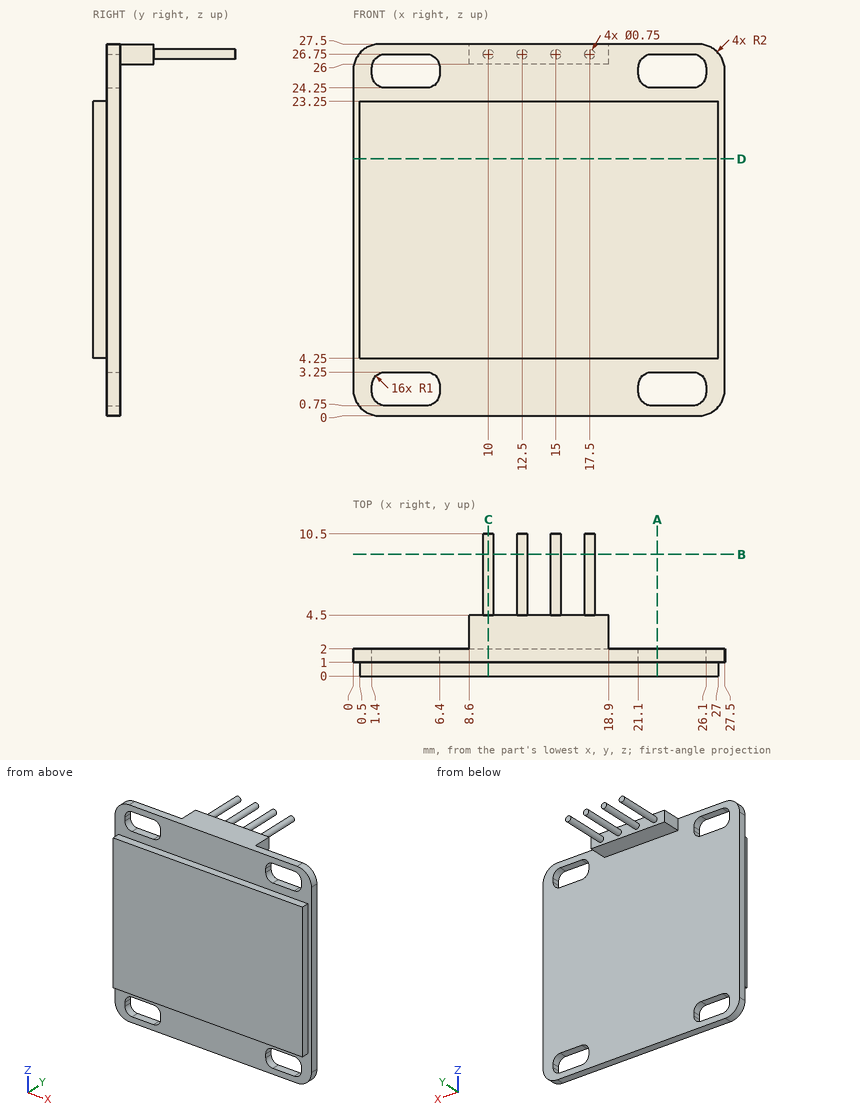
The drawing under review shows one solid part. Ordinate dimensions are in mm from its lowest x, y, z. Coordinates: 2 decimals unless noted, no trailing zeros. Write each loop counter-clockwise with the first axis right and the second up, starting at its lowest first coordinate (ties: lowest second). Pieces come first, ordered by that corner, then holes.
1) Insertion check: pin 1 (12 mm diameter, centred on x = 6.5, z = 3, fed in from +Y); pin 2 (0.5 mm diameter, centred on y = 0.5, z = 14, fed in from -X); pin 3 (0.5 mm diameter, centred on x = 11.5, y = 0.5, fed in from -Z). Each pin has a flat end and moves straight along its axis. Give the tip position at first contact, or say it passes through.
2) Add section A-A (x = 22.5). Write out the cut boundary in (y, z).
3) To check wall thickness, follow L1, parallel to Y at x = 19.75, z = 7; L2, parallel to Y at x = 20.5, z = 23.75; L3, parallel to Z at x = 8.75, y = 4.25. State the ranges of each line that lie inside material, in increasing order.
4) Add section D-D (z = 19). Write out the cut boundary in (x, y), plus the area to 3 significant figures.
5) Add section C-C (x = 10). Write out the cut boundary in (y, z) (3 decimals).
6) Add section B-B (y = 9). Write out the cut boundary in (x, z) (3 decimals), plus the area to 3 significant figures.
Check result:
1. pin 1: stops at y = 2
1. pin 2: stops at x = 0.5
1. pin 3: stops at z = 4.25
2. outline: (0, 4.25) - (1, 4.25) - (1, 3.25) - (2, 3.25) - (2, 24.25) - (1, 24.25) - (1, 23.25) - (0, 23.25) - close; (1, 0) - (2, 0) - (2, 0.75) - (1, 0.75) - close; (1, 26.75) - (2, 26.75) - (2, 27.5) - (1, 27.5) - close
3. L1: y = 0 to 2
3. L2: y = 1 to 2
3. L3: z = 26 to 27.5
4. outline: (0, 1) - (0.5, 1) - (0.5, 0) - (27, 0) - (27, 1) - (27.5, 1) - (27.5, 2) - (0, 2) - close
4. area: 54.0 mm2
5. outline: (0, 4.25) - (1, 4.25) - (1, 0) - (2, 0) - (2, 26) - (4.5, 26) - (4.5, 26.375) - (10.5, 26.375) - (10.5, 27.125) - (4.5, 27.125) - (4.5, 27.5) - (1, 27.5) - (1, 23.25) - (0, 23.25) - close
6. outline: circle Ø0.75 at (10, 26.75); circle Ø0.75 at (12.5, 26.75); circle Ø0.75 at (15, 26.75); circle Ø0.75 at (17.5, 26.75)
6. area: 1.77 mm2
